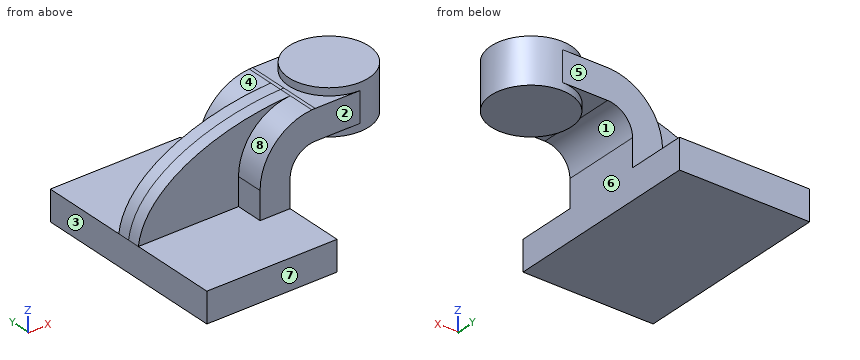
from build123d import *

# Parameters (mm, degrees)
F1_DEPTH = 63.5
F2_W     = 25.4
F2_H     = 19.05
F3_DEPTH = 25.4
F5_DEPTH = 7.9375


with BuildPart() as f1:
    # F0 (on Front) → F1 (new body, symmetric)
    with BuildSketch(Plane.XZ):
        Polygon((-41.275, 9.525), (-41.275, -9.525), (41.275, -9.525), (41.275, 9.525), (22.225, 9.525), align=None)
    extrude(amount=F1_DEPTH, both=True)

    # F2 (on face) + F0 (on Front) → F3 (join, symmetric)
    with BuildSketch(Plane.XZ):
        with Locations((73.025, 52.4002)):
            Rectangle(F2_W, F2_H)
    with BuildSketch(Plane.XZ):
        with BuildLine():
            Line((22.225, 9.525), (41.275, 9.525))
            Line((41.275, 9.525), (41.275, 27.0002))
            ThreePointArc((41.275, 27.0002), (45.9246798487, 38.2255201513), (57.15, 42.8752))
            Line((57.15, 42.8752), (60.325, 42.8752))
            Line((60.325, 42.8752), (60.325, 61.9252))
            Line((60.325, 61.9252), (57.15, 61.9252))
            add(Edge.make_bspline(
                [(55.0536793092, 61.8622289794), (55.7537102916, 61.8873697965), (56.452550575, 61.9083613576), (57.15, 61.9252)],
                knots=[109.7467015362, 109.7467015362, 109.7467015362, 109.7467015362, 111.5045361635, 111.5045361635, 111.5045361635, 111.5045361635], degree=3))
            ThreePointArc((55.0536793092, 61.8622289794), (31.7239343869, 50.9432744149), (22.225, 27.0002))
            Line((22.225, 27.0002), (22.225, 9.525))
        make_face()
    extrude(amount=F3_DEPTH, both=True)

    # F0 (on Front) → F5 (join, symmetric)
    with BuildSketch(Plane.XZ):
        with BuildLine():
            add(Edge.make_bspline(
                [(-41.275, 9.525), (-36.9974255187, 42.549756512), (11.3487197513, 60.2926150292), (55.0536793092, 61.8622289794)],
                knots=[0, 0, 0, 0, 109.7467015362, 109.7467015362, 109.7467015362, 109.7467015362], degree=3))
            Line((-41.275, 9.525), (22.225, 9.525))
            Line((22.225, 9.525), (22.225, 27.0002))
            ThreePointArc((22.225, 27.0002), (31.7239343869, 50.9432744149), (55.0536793092, 61.8622289794))
        make_face()
    extrude(amount=F5_DEPTH, both=True)

    # F6 (on face) → F7 (revolve)
    with BuildSketch(Plane.XZ):
        Polygon((111.125, 66.675), (85.725, 66.675), (85.725, 61.9252), (85.725, 42.8752), (85.725, 38.1), (111.125, 38.1), align=None)
    revolve(axis=Axis((85.725, 0, 52.3875), (0, 0, 1)))


solid = f1.part
Input: part model. Units: mm. Frame: model coordinates. Face numbers are marked on the shaded views. A direction names the side the tool comes from. Coordinates: 2 decimals unless noted, no trailing zeros. Loops run counter-clockwise (first coordinate to the right, second up) from the corner with the lowest first, then second, coordinate; pieces in that order, holes last. Notation, with made-up numbers: (10.25, 33) - (48.25, 33) arc R22 cw to (48.25, 57) - close; hole circle Ø3 at (46, 11). An arc over 180 degrees is marked (long way). Answer in a Markdown table with one row per item. Add a question column.
Item 1: Contact query for flat-ended pins moving along their axis: P1, Ø8.5, axis at y = -17, z = 15, coming from the -X side (3 decimals); P2, Ø15.5, axis at x = 54.5, z = 27.5, coming from the -Y side; P3, Ø4, axis at x = 46, y = 3.5, coming from the +Z side; P4, Ø8, axis at y = 0.5, z = 25.5, coming from the -X side. Output: stop coordinate, or through.
Item 2: Mould query, pull axis X, two halves, no side actions, for the marked faces 1, 2 and 3. Classes: released by +X, released by -X, zero draft, split by the parting line, or undercut.
Item 3: Access query for the marked faces 4, 5, 6, 7 and 8. Directions: +Z, -Z, +X, -X, +Y, -Y. A direction counts if a zero-diameter tool reaches every point of the face in a straight line with its end or side. Return the directions, or none.
Item 4: Section query A-A on z = 2. Return the cut outline in (x, y) (3 decimals).
Item 5: Line query: line 1 along Z through (x, y) = (85, -5) (3 decimals); line 2 along Z through (x, y) = (-21.5, 50) (3 decimals); line 3 along X through (y, z) = (-3, 4.5) (3 decimals). Output: solid intervals per line, ascending. Write a range as [from, to].
Item 6: Section query B-B on y = 34. Return the cut outline in (x, z) (3 decimals).
Recorded:
| question | item | result |
|---|---|---|
| 1 | P1 | x = 22.225 |
| 1 | P2 | through |
| 1 | P3 | z = 61.47 |
| 1 | P4 | x = -37.54 |
| 2 | face 1 | undercut |
| 2 | face 2 | zero draft |
| 2 | face 3 | released by -X |
| 3 | face 4 | +Z, -X, +Y |
| 3 | face 5 | +Z, +X, -X, +Y |
| 3 | face 6 | -Z, +X, +Y, -Y |
| 3 | face 7 | +Z, -Z, +X, -X, -Y |
| 3 | face 8 | +Z, -X, -Y |
| 4 | outline | (-41.275, -63.5) - (41.275, -63.5) - (41.275, 63.5) - (-41.275, 63.5) - close |
| 5 | line 1 | [38.1, 66.675] |
| 5 | line 2 | [-9.525, 9.525] |
| 5 | line 3 | [-41.275, 41.275] |
| 6 | outline | (-41.275, -9.525) - (41.275, -9.525) - (41.275, 9.525) - (-41.275, 9.525) - close |
